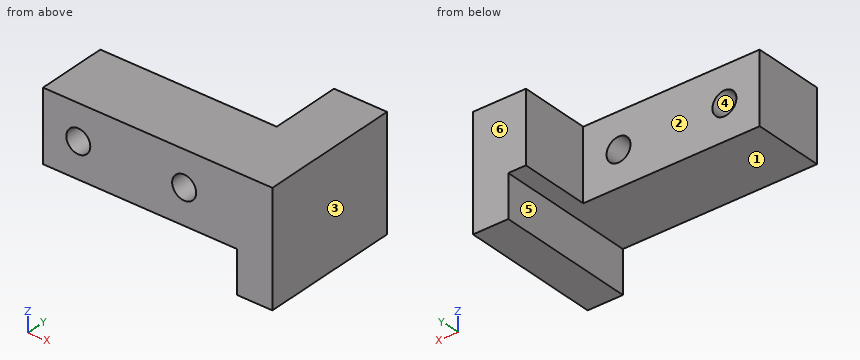
from build123d import *

# Parameters (mm, degrees)
SKETCH1_W           = 25
SKETCH1_H           = 10
SKETCH1_R           = 1.7
BOSS_EXTRUDE1_DEPTH = 10
BOSS_EXTRUDE2_DEPTH = 20


with BuildPart() as part:
    # Sketch1 → Boss-Extrude1 (new body)
    with BuildSketch(Plane(origin=(0, 0, 0), x_dir=(1, 0, 0), z_dir=(0, 1, 0))):
        Rectangle(SKETCH1_W, SKETCH1_H)
        with Locations(Location((-7.5, 0, 0), (0, 0, 270))):
            Circle(SKETCH1_R, mode=Mode.SUBTRACT)
        with Locations(Location((7.5, 0, 0), (0, 0, 270))):
            Circle(SKETCH1_R, mode=Mode.SUBTRACT)
    extrude(amount=BOSS_EXTRUDE1_DEPTH)

    # Sketch2 → Boss-Extrude2 (add)
    with BuildSketch(Plane(origin=(0, 0, 0), x_dir=(1, 0, 0), z_dir=(0, 1, 0))):
        Polygon((12.5, -5), (20, -5), (20, 11), (15, 11), (15, 5), (12.5, 5), align=None)
    extrude(amount=BOSS_EXTRUDE2_DEPTH)


solid = part.part
Input: part model. Units: mm. Frame: model coordinates. Face numbers are marked on the shaded views. A direction names the side the tool comes from. Coordinates: 2 decimals unless noted, no trailing zeros. Order: outer loops, then holes, each group sorted by start corner. A loop starts at its lowest first (then second) coordinate and runs counter-clockwise, first axis right, second up. Notation, with made-up numbers: M 81,0 L 135,0 A8 ccw 135,12 Z; hole C -4.5,26 d8. An arc over 180 degrees is marked long. One line per question, with ' | ' between items.
Item 1: Pin query (flat end, axial travel): pin 1 (1 mm diameter, centred on x = 1.5, y = 10, fed in from -Z); pin 2 (8 mm diameter, centred on y = 17, z = 0, fed in from -X); pin 3 (4 mm diameter, centred on x = 11.5, z = -6, fed in from +Y); pin 4 (5 mm diameter, centred on x = -3.5, z = -2, fed in from +Y). Return the tip coordinate at first contact, or that it passes through.
Geometry results:
pin 1: stops at z = -5 | pin 2: stops at x = 12.5 | pin 3: stops at y = 20 | pin 4: stops at y = 10
Item 2: Section B-B (x = 7.5). Output: boundary loops of the cut face in (y, z).
Geometry results:
outline: M 0,-5 L 10,-5 L 10,-1.7 L 0,-1.7 Z; M 0,1.7 L 10,1.7 L 10,5 L 0,5 Z
Item 3: Section A-A (z = 0). Output: boundary loops of the cut face in (x, y).
Geometry results:
outline: M -12.5,0 L -9.2,0 L -9.2,10 L -12.5,10 Z; M -5.8,0 L 5.8,0 L 5.8,10 L -5.8,10 Z; M 9.2,0 L 20,0 L 20,20 L 12.5,20 L 12.5,10 L 9.2,10 Z
Item 4: Ray query, line 1 along X through (y, z) = (3, 0); line 2 along Z through (x, y) = (-10, 7.25); line 3 along X through (y, z) = (13.75, -1.25). Return the intervals inside material, ascending.
Geometry results:
line 1: x = -12.5 to -9.2, -5.8 to 5.8, 9.2 to 20 | line 2: z = -5 to 5 | line 3: x = 12.5 to 20
Item 5: Draft query along X for the marked faces 4, 5 and 6. Return one class per face: released by +X, released by -X, zero draft, split by the parting line, or undercut.
Geometry results:
face 4: undercut | face 5: released by -X | face 6: zero draft
Item 6: Section C-C (y = 3). Output: boundary loops of the cut face in (x, z), then the cut area to 3 significant figures.
Geometry results:
outline: M -12.5,-5 L 15,-5 L 15,-11 L 20,-11 L 20,5 L -12.5,5 Z; hole C -7.5,0 d3.4; hole C 7.5,0 d3.4 | area: 337 mm^2
Item 7: Section D-D (z = -3.75). Output: boundary loops of the cut face in (x, y).
Geometry results:
outline: M -12.5,0 L 20,0 L 20,20 L 12.5,20 L 12.5,10 L -12.5,10 Z
Item 8: Reachability of the marked faces 1, 2 and 3 from +Z, -Z, +X, -X, +Y, -Y: full face, straight path, thin tool, end or side. Return the list, or none.
Geometry results:
face 1: -Z, -X, +Y, -Y | face 2: +Z, -Z, -X, +Y | face 3: +Z, -Z, +X, +Y, -Y
